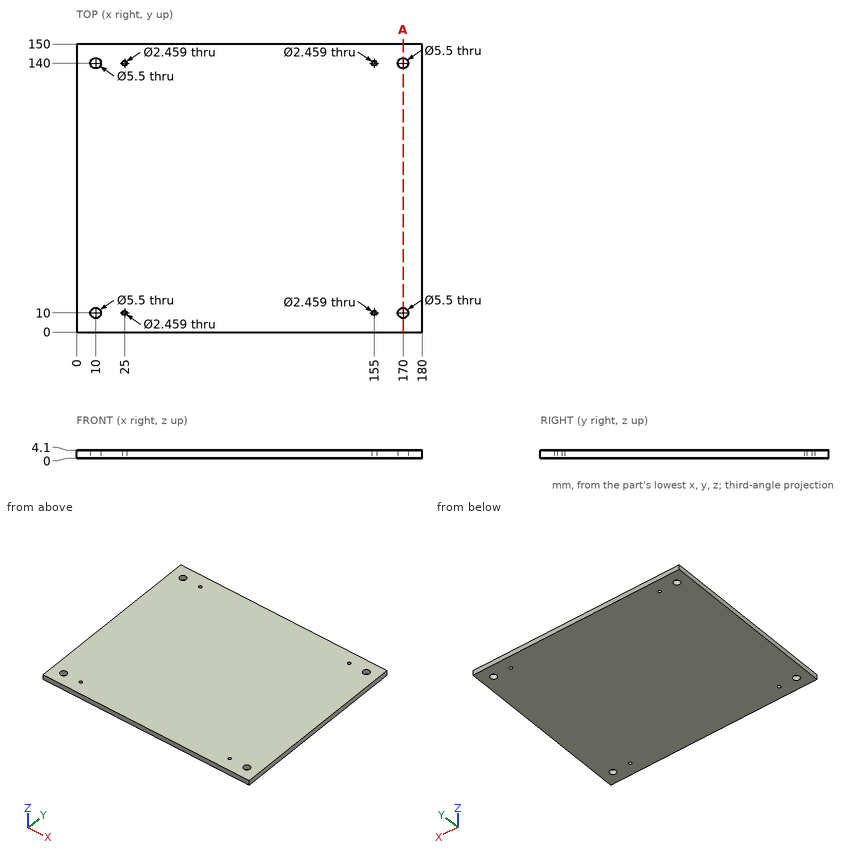
Study the drawing (mm; zero at the part's minimum x, y, z) and answer. Round coordinates to 2 decimals unless told otherwise and drop trailing zeros. Write each loop counter-clockwise with the first axis right and the second up, starting at its lowest first coordinate (ties: lowest second). Pieces come first, ordered by that corner, then holes. Notation, with made-up numbers: (51, 82.5) - (61, 82.5) arc R23 ccw to (61, 118.5) - close; hole circle Ø8 at (-8, 87.5). An arc over 180 degrees is marked (long way). Use a Markdown table: item, result. Add a question column.
1. Consider line 1 (Y direction, x = 170, z = 1.6); line 2 (X direction, y = 140, z = 2.9); line 3 (Y direction, x = 25, z = 3.05). Determine where each line is inside the solid, lowest interval first.
2. The part is cut by section A-A (x = 170). Write down the section's boundary in (y, z).
3. A flat-ended cylindrical pin translates along its axis: P1, Ø4.5, axis at x = 10, y = 140, coming from the +Z side. Find the tip coordinate at first contact, or state that the pin passes through.
Reported:
| question | item | result |
|---|---|---|
| 1 | line 1 | 0 to 7.25, 12.75 to 137.25, 142.75 to 150 |
| 1 | line 2 | 0 to 7.25, 12.75 to 23.77, 26.23 to 153.77, 156.23 to 167.25, 172.75 to 180 |
| 1 | line 3 | 0 to 8.77, 11.23 to 138.77, 141.23 to 150 |
| 2 | outline | (0, 0) - (7.25, 0) - (7.25, 4.1) - (0, 4.1) - close; (12.75, 0) - (137.25, 0) - (137.25, 4.1) - (12.75, 4.1) - close; (142.75, 0) - (150, 0) - (150, 4.1) - (142.75, 4.1) - close |
| 3 | P1 | through |
